from build123d import *

# Parameters (mm, degrees)
F1_W         = 72
F1_H         = 141
F2_DEPTH     = 8
F0_R         = 1
F3_DEPTH     = 0.2
F0_W         = 64
F0_H         = 113
F0_W_2       = 17
F0_H_2       = 1.5
F0_R_2       = 0.5
F4_DEPTH     = 0.2
F5_DEPTH     = 0.5
F1_R         = 1
F6_DEPTH     = 2
F0_W_3       = 16
F0_H_3       = 5
F7_DEPTH     = 0.5
F8_T1_DEPTH  = 77
F8_T3_DEPTH  = 146
F8_T5_DEPTH  = 16
F8_T7_DEPTH  = 5
F8_T13_DEPTH = 7.1650635095
F8_T17_DEPTH = 18.1650635095
F8_T24_DEPTH = 18.1650635095
F8_T28_DEPTH = 7.1650635095
F8_T35_DEPTH = 7.1650635095
F8_T39_DEPTH = 18.1650635095
F8_T46_DEPTH = 7.1650635095
F8_T50_DEPTH = 18.1650635095


# Not quite as in the source:
# - a fillet or chamfer that OpenCascade refuses, or shapes differently, is made with other operations: its cross-section is extruded or revolved along the edge and cut away or added


with BuildPart() as f2:
    # F1 (on face) → F2 (new body)
    with BuildSketch(Plane.XY):
        with Locations((-0.0423140228, 0.0165017247)):
            Rectangle(F1_W, F1_H)
    extrude(amount=-F2_DEPTH)

    # F0 (on Top) → F3 (cut)
    with BuildSketch(Plane.XY):
        with Locations((-23, 66.5)):
            Circle(F0_R)
        with Locations((13.5, 64.5)):
            Circle(F0_R)
        with Locations((16.5, 64.5)):
            Circle(F0_R)
    extrude(amount=-F3_DEPTH, mode=Mode.SUBTRACT)

    # F0 (on Top) → F4 (cut)
    with BuildSketch(Plane.XY):
        Rectangle(F0_W, F0_H)
        with Locations((0, 66.2368237972)):
            Rectangle(F0_W_2, F0_H_2)
        with Locations((-7.8863224118, 66.2359703599)):
            Circle(F0_R_2, mode=Mode.SUBTRACT)
        with Locations((-6.75, 66.25)):
            Circle(F0_R_2, mode=Mode.SUBTRACT)
        with Locations((-5.5, 66.25)):
            Circle(F0_R_2, mode=Mode.SUBTRACT)
        with Locations((-4.25, 66.2368237972)):
            Circle(F0_R_2, mode=Mode.SUBTRACT)
        with Locations((-3, 66.25)):
            Circle(F0_R_2, mode=Mode.SUBTRACT)
        with Locations((-1.75, 66.25)):
            Circle(F0_R_2, mode=Mode.SUBTRACT)
        with BuildLine():
            ThreePointArc((0, 65.7368237972), (-0.3535533906, 66.5903771878), (0.5, 66.2368237972))
            ThreePointArc((0.5, 66.2368237972), (0.3535533906, 65.8832704066), (0, 65.7368237972))
        make_face(mode=Mode.SUBTRACT)
        with Locations((1.75, 66.25)):
            Circle(F0_R_2, mode=Mode.SUBTRACT)
        with Locations((3, 66.25)):
            Circle(F0_R_2, mode=Mode.SUBTRACT)
        with Locations((4.25, 66.2368237972)):
            Circle(F0_R_2, mode=Mode.SUBTRACT)
        with Locations((5.5, 66.25)):
            Circle(F0_R_2, mode=Mode.SUBTRACT)
        with Locations((6.75, 66.25)):
            Circle(F0_R_2, mode=Mode.SUBTRACT)
        with Locations((7.8863224118, 66.2359703599)):
            Circle(F0_R_2, mode=Mode.SUBTRACT)
    extrude(amount=-F4_DEPTH, mode=Mode.SUBTRACT)

    # F0 (on Top) → F5 (cut)
    with BuildSketch(Plane.XY):
        with Locations((-7.8863224118, 66.2359703599)):
            Circle(F0_R_2)
        with Locations((-6.75, 66.25)):
            Circle(F0_R_2)
        with Locations((1.75, 66.25)):
            Circle(F0_R_2)
        with Locations((3, 66.25)):
            Circle(F0_R_2)
        with BuildLine():
            ThreePointArc((0, 65.7368237972), (0.3535533906, 65.8832704066), (0.5, 66.2368237972))
            ThreePointArc((0.5, 66.2368237972), (-0.3535533906, 66.5903771878), (0, 65.7368237972))
        make_face()
        with Locations((-4.25, 66.2368237972)):
            Circle(F0_R_2)
        with Locations((-3, 66.25)):
            Circle(F0_R_2)
        with Locations((-1.75, 66.25)):
            Circle(F0_R_2)
        with Locations((4.25, 66.2368237972)):
            Circle(F0_R_2)
        with Locations((5.5, 66.25)):
            Circle(F0_R_2)
        with Locations((6.75, 66.25)):
            Circle(F0_R_2)
        with Locations((7.8863224118, 66.2359703599)):
            Circle(F0_R_2)
        with Locations((-5.5, 66.25)):
            Circle(F0_R_2)
    extrude(amount=-F5_DEPTH, mode=Mode.SUBTRACT)

    # F1 (on face) → F6 (cut)
    with BuildSketch(Plane.XY):
        with Locations((26.0005407035, 63.5057538748)):
            Circle(F1_R)
    extrude(amount=-F6_DEPTH, mode=Mode.SUBTRACT)

    # F0 (on Top) → F7 (cut)
    with BuildSketch(Plane.XY):
        with Locations((0, -63)):
            Rectangle(F0_W_3, F0_H_3)
    extrude(amount=-F7_DEPTH, mode=Mode.SUBTRACT)

    # F8: fillet of radius 1 on 8 edges, made by hand

    # F8_s2 → F8_t1 (cut)
    with BuildSketch(Plane.YZ.offset(-38.5423140228)):
        with BuildLine():
            ThreePointArc((70.5165017247, -1), (70.2236085059, -0.2928932188), (69.5165017247, 0))
            Line((69.5165017247, 0), (70.5165017247, 0))
            Line((70.5165017247, 0), (70.5165017247, -1))
        make_face()
        with BuildLine():
            ThreePointArc((-70.4834982753, -1), (-70.1906050565, -0.2928932188), (-69.4834982753, 0))
            Line((-69.4834982753, 0), (-70.4834982753, 0))
            Line((-70.4834982753, 0), (-70.4834982753, -1))
        make_face()
    extrude(amount=F8_T1_DEPTH, mode=Mode.SUBTRACT)

    # F8_s4 → F8_t3 (cut)
    with BuildSketch(Plane.XZ.offset(-73.0165017247)):
        with BuildLine():
            ThreePointArc((-35.0423140228, 0), (-35.749420804, -0.2928932188), (-36.0423140228, -1))
            Line((-36.0423140228, -1), (-36.0423140228, 0))
            Line((-36.0423140228, 0), (-35.0423140228, 0))
        make_face()
        with BuildLine():
            ThreePointArc((35.9576859772, -1), (35.6647927584, -0.2928932188), (34.9576859772, 0))
            Line((34.9576859772, 0), (35.9576859772, 0))
            Line((35.9576859772, 0), (35.9576859772, -1))
        make_face()
    extrude(amount=F8_T3_DEPTH, mode=Mode.SUBTRACT)

    # F8_s6 → F8_t5 (cut)
    with BuildSketch(Plane.YZ.offset(-8)):
        with BuildLine():
            ThreePointArc((-59.6339745962, 0), (-60.1339745962, -0.1339745962), (-60.5, -0.5))
            Line((-60.5, -0.5), (-60.5, 0))
            Line((-60.5, 0), (-59.6339745962, 0))
        make_face()
        with BuildLine():
            ThreePointArc((-66.3660254038, 0), (-65.8660254038, -0.1339745962), (-65.5, -0.5))
            Line((-65.5, -0.5), (-65.5, 0))
            Line((-65.5, 0), (-66.3660254038, 0))
        make_face()
    extrude(amount=F8_T5_DEPTH, mode=Mode.SUBTRACT)

    # F8_s8 → F8_t7 (cut)
    with BuildSketch(Plane.XZ.offset(60.5)):
        with BuildLine():
            ThreePointArc((-8.8660254038, 0), (-8.3660254038, -0.1339745962), (-8, -0.5))
            Line((-8, -0.5), (-8, 0))
            Line((-8, 0), (-8.8660254038, 0))
        make_face()
        with BuildLine():
            ThreePointArc((8.8660254038, 0), (8.3660254038, -0.1339745962), (8, -0.5))
            Line((8, -0.5), (8, 0))
            Line((8, 0), (8.8660254038, 0))
        make_face()
    extrude(amount=F8_T7_DEPTH, mode=Mode.SUBTRACT)


with BuildPart() as f8_tool11:
    # F8_s12 → F8_t13 (new body)
    with BuildSketch(Plane.XZ.offset(65.5)):
        with BuildLine():
            ThreePointArc((8.8660254038, 0), (8.3660254038, -0.1339745962), (8, -0.5))
            Line((8, -0.5), (8, 0))
            Line((8, 0), (8.8660254038, 0))
        make_face()
    extrude(amount=-F8_T13_DEPTH)

    split(bisect_by=Plane.XZ.offset(60.5), keep=Keep.BOTTOM)


with BuildPart() as f8_tool15:
    # F8_s16 → F8_t17 (new body)
    with BuildSketch(Plane.YZ.offset(10.1650635095)):
        with BuildLine():
            ThreePointArc((-59.6339745962, 0), (-60.1339745962, -0.1339745962), (-60.5, -0.5))
            Line((-60.5, -0.5), (-60.5, 0))
            Line((-60.5, 0), (-59.6339745962, 0))
        make_face()
    extrude(amount=-F8_T17_DEPTH)

    split(bisect_by=Plane.YZ.offset(8), keep=Keep.TOP)


with BuildPart() as f8_tool11_1:
    add(f8_tool11.part)

    # F8_t19: intersect F8_tool15
    add(f8_tool15.part, mode=Mode.INTERSECT)


with BuildPart() as f2_1:
    add(f2.part)

    # F8_t9: cut F8_tool11
    add(f8_tool11_1.part, mode=Mode.SUBTRACT)


with BuildPart() as f8_tool22:
    # F8_s23 → F8_t24 (new body)
    with BuildSketch(Plane.YZ.offset(8)):
        with BuildLine():
            ThreePointArc((-59.6339745962, 0), (-60.1339745962, -0.1339745962), (-60.5, -0.5))
            Line((-60.5, -0.5), (-60.5, 0))
            Line((-60.5, 0), (-59.6339745962, 0))
        make_face()
    extrude(amount=-F8_T24_DEPTH)

    split(bisect_by=Plane.YZ.offset(-8), keep=Keep.BOTTOM)


with BuildPart() as f8_tool26:
    # F8_s27 → F8_t28 (new body)
    with BuildSketch(Plane.XZ.offset(58.3349364905)):
        with BuildLine():
            ThreePointArc((-8.8660254038, 0), (-8.3660254038, -0.1339745962), (-8, -0.5))
            Line((-8, -0.5), (-8, 0))
            Line((-8, 0), (-8.8660254038, 0))
        make_face()
    extrude(amount=F8_T28_DEPTH)

    split(bisect_by=Plane.XZ.offset(60.5), keep=Keep.BOTTOM)


with BuildPart() as f8_tool22_1:
    add(f8_tool22.part)

    # F8_t30: intersect F8_tool26
    add(f8_tool26.part, mode=Mode.INTERSECT)


with BuildPart() as f2_2:
    add(f2_1.part)

    # F8_t20: cut F8_tool22
    add(f8_tool22_1.part, mode=Mode.SUBTRACT)


with BuildPart() as f8_tool33:
    # F8_s34 → F8_t35 (new body)
    with BuildSketch(Plane.XZ.offset(60.5)):
        with BuildLine():
            ThreePointArc((-8.8660254038, 0), (-8.3660254038, -0.1339745962), (-8, -0.5))
            Line((-8, -0.5), (-8, 0))
            Line((-8, 0), (-8.8660254038, 0))
        make_face()
    extrude(amount=F8_T35_DEPTH)

    split(bisect_by=Plane.XZ.offset(65.5), keep=Keep.TOP)


with BuildPart() as f8_tool37:
    # F8_s38 → F8_t39 (new body)
    with BuildSketch(Plane.YZ.offset(-10.1650635095)):
        with BuildLine():
            ThreePointArc((-66.3660254038, 0), (-65.8660254038, -0.1339745962), (-65.5, -0.5))
            Line((-65.5, -0.5), (-65.5, 0))
            Line((-65.5, 0), (-66.3660254038, 0))
        make_face()
    extrude(amount=F8_T39_DEPTH)

    split(bisect_by=Plane.YZ.offset(-8), keep=Keep.BOTTOM)


with BuildPart() as f8_tool33_1:
    add(f8_tool33.part)

    # F8_t41: intersect F8_tool37
    add(f8_tool37.part, mode=Mode.INTERSECT)


with BuildPart() as f2_3:
    add(f2_2.part)

    # F8_t31: cut F8_tool33
    add(f8_tool33_1.part, mode=Mode.SUBTRACT)


with BuildPart() as f8_tool44:
    # F8_s45 → F8_t46 (new body)
    with BuildSketch(Plane.XZ.offset(67.6650635095)):
        with BuildLine():
            ThreePointArc((8.8660254038, 0), (8.3660254038, -0.1339745962), (8, -0.5))
            Line((8, -0.5), (8, 0))
            Line((8, 0), (8.8660254038, 0))
        make_face()
    extrude(amount=-F8_T46_DEPTH)

    split(bisect_by=Plane.XZ.offset(65.5), keep=Keep.TOP)


with BuildPart() as f8_tool48:
    # F8_s49 → F8_t50 (new body)
    with BuildSketch(Plane.YZ.offset(-8)):
        with BuildLine():
            ThreePointArc((-66.3660254038, 0), (-65.8660254038, -0.1339745962), (-65.5, -0.5))
            Line((-65.5, -0.5), (-65.5, 0))
            Line((-65.5, 0), (-66.3660254038, 0))
        make_face()
    extrude(amount=F8_T50_DEPTH)

    split(bisect_by=Plane.YZ.offset(8), keep=Keep.TOP)


with BuildPart() as f8_tool44_1:
    add(f8_tool44.part)

    # F8_t52: intersect F8_tool48
    add(f8_tool48.part, mode=Mode.INTERSECT)


with BuildPart() as f2_4:
    add(f2_3.part)

    # F8_t42: cut F8_tool44
    add(f8_tool44_1.part, mode=Mode.SUBTRACT)


solid = f2_4.part
Model file for the job. Use its own axes, mm. A direction names the side the tool comes from. Give positions to 0.01 mm unless a question says otherwise; leave off trailing zeros. Order: outer loops, then holes, each group sorted by start corner. A loop starts at its lowest first (then second) coordinate and runs counter-clockwise, first axis right, second up. Notation, with made-up numbers: M 57,-28 L 75,-28 A25 cw 75,-11 Z; hole C 32.25,70.5 d3. An arc over 180 degrees is marked long. Put each result on its own line as item: value. Start each with the question number.
(1) Pin check, flat tips, straight feed: pin 1 Ø0.8 at (x, y) = (0, 66) entering from +Z; pin 2 Ø1.5 at (x, y) = (-4, -62.5) entering from +Z. Stop position of each tip, or through.
(2) Tool access for faces 4 (the face through (0, 1, -0.2)), 5 (the face through (-34, 11, 0)): list every direction of +Z, -Z, +X, -X, +Y, -Y with a clear straight run to the whole face (end or side of a thin tool).
(3) Band-saw the part on A-A on y = -49. Give the cut face in (x, z), then the cut area to 3 significant figures.
(4) Drill centre lines: L1, parallel to Y at x = 0, z = -0.25; L2, parallel to Y at x = 16.5, z = -0.1; L3, parallel to Z at x = 10, y = 17. Where is each one in solid material? Low to high. Write a range as [from, to].
(5) Pull direction X, two halves, no side cores. Call faces 1 (the face through (-36.042, -1, -4)), 2 (the face through (-1, 70.517, -4)), 3 (the face through (0, -63, -0.5)): released by +X, released by -X, zero draft, split by the parting line, or undercut.
Results below:
1. pin 1: stops at z = -0.2
1. pin 2: stops at z = -0.5
2. face 4: +Z
2. face 5: +Z, +X, -X, +Y, -Y
3. outline: M -36.04,-8 L 35.96,-8 L 35.96,-1 A1 ccw 34.96,0 L 32,0 L 32,-0.2 L -32,-0.2 L -32,0 L -35.04,0 A1 ccw -36.04,-1 Z
3. area: 563 mm2
4. L1: y = [-70.14, -65.7], [-60.3, 65.74], [66.74, 70.18]
4. L2: y = [-69.92, -56.5], [56.5, 63.5], [65.5, 69.95]
4. L3: z = [-8, -0.2]
5. face 1: released by -X
5. face 2: zero draft
5. face 3: undercut
